```python
from build123d import *

# Parameters (mm, degrees)
F2_W          = 80
F2_H          = 80
F3_DEPTH      = 40
F7_ANGLE_BACK = 35
F7_ANGLE      = 70
F8_R          = 3
F9_DEPTH      = 4
F10_R         = 10
F11_DEPTH     = 5
F12_R         = 10
F13_DEPTH     = 5


# Not quite as in the source:
# - a feature names something its author has since deleted; it is built from what else it names


with BuildPart() as f1:
    # F0 (on Top) → F1 (revolve)
    with BuildSketch(Plane.XY):
        with BuildLine():
            Line((0, 37), (0, -37))
            ThreePointArc((0, -37), (37, 0), (0, 37))
        make_face()
    revolve(axis=Axis((0, 0, 0), (0, -1, 0)))


with BuildPart() as f3:
    # F2 (on Top) → F3 (new body, symmetric)
    with BuildSketch(Plane.XY):
        Rectangle(F2_W, F2_H)
    extrude(amount=F3_DEPTH, both=True)

    # F4: cut F1
    add(f1.part, mode=Mode.SUBTRACT)

    # F6 (on Front) → F7 (revolve)
    with BuildSketch(Plane.XZ, mode=Mode.PRIVATE) as f7_sk:
        with BuildLine():
            add(Edge.make_bspline(
                [(-28.4972605327, -23.5988589159), (-22.613415631, -15.226576282), (-15.2284997687, -1.2521191935), (-21.0733372873, 17.730814669), (-28.4972605327, 23.5988589159)],
                knots=[0, 0, 0, 0, 0.5, 1, 1, 1, 1], degree=3))
            ThreePointArc((-28.4972605327, 23.5988589159), (-29.0776083413, 22.8799626999), (-29.6398253299, 22.1468000942))
            add(Edge.make_bspline(
                [(-29.6398253299, 22.1468000942), (-23.6962903291, 15.970768407), (-17.3082405815, -0.7806496907), (-24.5547182858, -14.3142519519), (-29.8117857382, -21.9147765469)],
                knots=[0, 0, 0, 0, 0.5007860737, 1, 1, 1, 1], degree=3))
            ThreePointArc((-29.8117857382, -21.9147765469), (-29.1666805209, -22.7663072849), (-28.4972605327, -23.5988589159))
        make_face()
    revolve(f7_sk.sketch.rotate(Axis((-40, 0, 0), (0, 0, -1)), -F7_ANGLE_BACK), axis=Axis((-40, 0, 0), (0, 0, -1)), revolution_arc=F7_ANGLE)

    # F8 (on face) → F9 (cut, symmetric)
    with BuildSketch(Plane(origin=(-40, 0, 0), x_dir=(0, -1, 0), z_dir=(-1, 0, 0))):
        Circle(F8_R)
    extrude(amount=F9_DEPTH, both=True, mode=Mode.SUBTRACT)

    # F10 (on face) → F11 (cut, symmetric)
    with BuildSketch(Plane.XY.offset(40)):
        Circle(F10_R)
    extrude(amount=F11_DEPTH, both=True, mode=Mode.SUBTRACT)

    # F12 (on face) → F13 (cut, symmetric)
    with BuildSketch(Plane(origin=(0, 0, -40), x_dir=(1, 0, 0), z_dir=(0, 0, -1))):
        Circle(F12_R)
    extrude(amount=F13_DEPTH, both=True, mode=Mode.SUBTRACT)


solid = f3.part
```
Check sheet for the modelled part. Datum: model origin and axes. Units: mm. A direction names the side the tool comes from. Coordinates: 2 decimals unless noted, no trailing zeros. Loops run counter-clockwise (first coordinate to the right, second up) from the corner with the lowest first, then second, coordinate; pieces in that order, holes last. Notation, with made-up numbers: M 39,26 L 84,26 A16 cw 84,38 Z; hole C 56,80 d4. An arc over 180 degrees is marked long. Answer as a JSON object with one key per item and string values.
1. Sectioned sample at C-C on y = -25.5. Record the cut outline in (x, z), and give its area (3 significant figures).
Outcome:
{"outline": "M -40,-40 L 40,-40 L 40,40 L -40,40 Z; hole C 0,0 d53.62", "area": "4,140 mm²"}
2. Release check for a two-part mould opening along Y. For faces 3 (the flat face through (-1, -40, 1)), 4 (the flat face through (-9, -8, 40)), 5 (the flat face through (-1, 40, 1)), 6 (the cylindrical face through (-38, 3, 0)) record: pulls with the +Y half, pulls with the -Y half, needs draft (parallel to the pull), parting line crosses it, or undercut.
Outcome:
{"face 3": "pulls with the -Y half", "face 4": "needs draft", "face 5": "pulls with the +Y half", "face 6": "undercut"}
3. Sectioned sample at B-B on z = 30.5. Record the cut outline in (x, y).
Outcome:
{"outline": "M -40,-40 L 40,-40 L 40,40 L -40,40 Z; hole C 0,0 d41.89"}
4. Sectioned sample at D-D on x = -8.5. Record the cut outline in (y, z), and give its area (3 significant figures).
Outcome:
{"outline": "M -40,-40 L -5.27,-40 L -5.27,-35.62 A36.01 cw -5.27,35.62 L -5.27,40 L -40,40 Z; M 5.27,-40 L 40,-40 L 40,40 L 5.27,40 L 5.27,35.62 A36.01 cw 5.27,-35.62 Z", "area": "2,240 mm²"}
5. Access from +Z, -Z, +X, -X, +Y, -Y to the whole of each face (thin tool, end or side, straight path). Record for faces 1 (the flat face through (-23.85, -11.31, 0.32)), 2 (the cylindrical face through (-2.17, -9.76, 37.84)).
Outcome:
{"face 1": "none", "face 2": "+Z, -Z"}
6. Scan lines: L1, parallel to X at y = 0, z = -37.4; L2, parallel to Z at x = -38, y = 0. Record each from-to range of solid material in increasing order. Write a range as from..to.
Outcome:
{"L1": "-40..-10, 10..40", "L2": "-40..-3, 3..40"}
7. Depth check by flat-ended pin: P1, Ø12, axis at x = -1, y = 8.5, coming from the -Z side; P2, Ø16, axis at x = 0, y = 0, coming from the +Z side. Enter the tip coordinate at first touch or a pass-through.
Outcome:
{"P1": "z = -40", "P2": "through"}
8. Sectioned sample at A-A on x = 0. Record the cut outline in (y, z), and give its area (3 significant figures).
Outcome:
{"outline": "M -40,-40 L -10,-40 L -10,-35.62 A37 cw -10,35.62 L -10,40 L -40,40 Z; M 10,-40 L 40,-40 L 40,40 L 10,40 L 10,35.62 A37 cw 10,-35.62 Z", "area": "1,960 mm²"}
